Drawing for the job (mm, zero at the part's lowest x, y, z). A direction names the side the tool comes from. Coordinates: 2 decimals unless noted, no trailing zeros. Loops run counter-clockwise (first coordinate to the right, second up) from the corner with the lowest first, then second, coordinate; pieces in that order, holes last. Notation, with made-up numbers: (28.25, 8) -> (66.25, 8) arc R20 ccw to (66.25, 26) -> close; hole circle Ø1 at (72.25, -29). An arc over 180 degrees is marked (long way). Write each question's results on one line, items separated by ' | '.
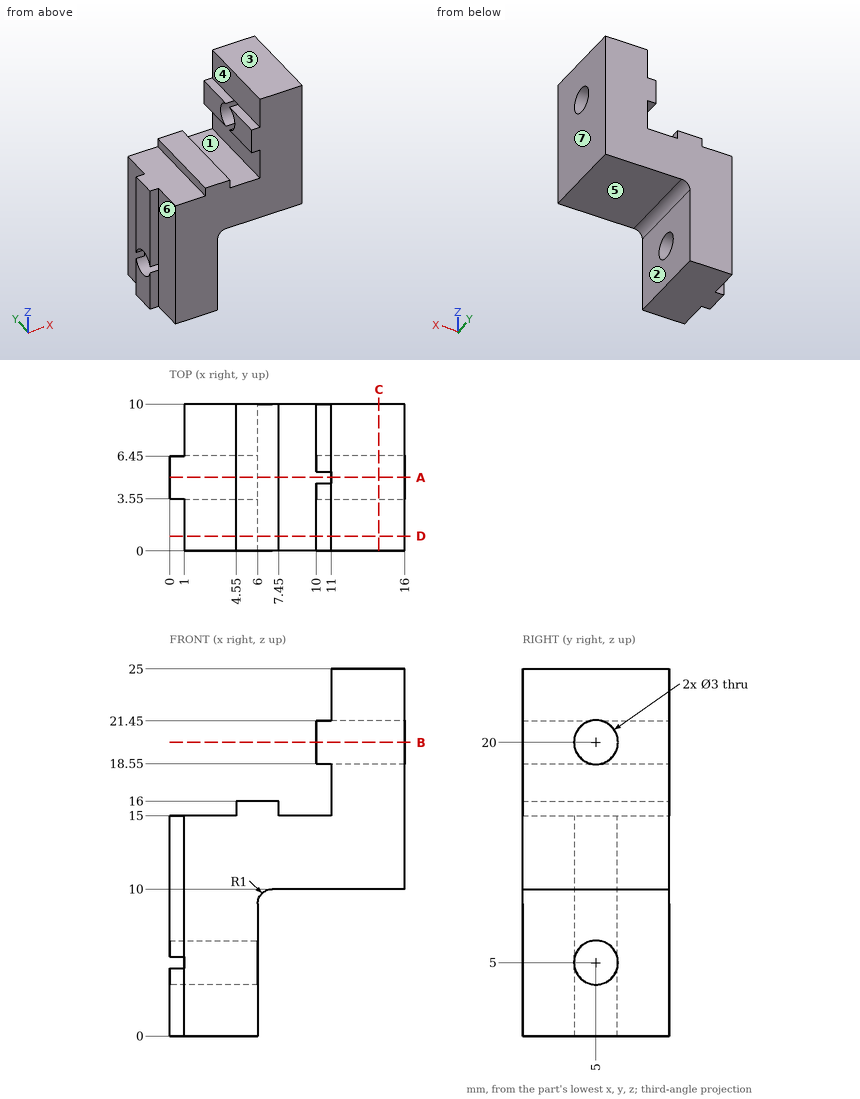
1) Slice it at D-D (y = 1). Write the cut outline in (x, z).
Outcome:
outline: (1, 0) -> (6, 0) -> (6, 9) arc R1 cw to (7, 10) -> (16, 10) -> (16, 25) -> (11, 25) -> (11, 21.45) -> (10, 21.45) -> (10, 18.55) -> (11, 18.55) -> (11, 15) -> (7.45, 15) -> (7.45, 16) -> (4.55, 16) -> (4.55, 15) -> (1, 15) -> close
2) Two-plate mould, pull along X, no slides. Class the marked faces 1, 2 and 3: pulls with the +X half, pulls with the -X half, needs draft (parallel to the pull), parting line crosses it, or undercut.
Outcome:
face 1: undercut | face 2: pulls with the +X half | face 3: needs draft
3) Drill centre lines: L1, parallel to Y at x = 12.7, z = 20; L2, parallel to Z at x = 3.65, y = 5; L3, parallel to Z at x = 14.15, y = 5. Where is each one in solid material? Low to high. Write a range as from..to.
Outcome:
L1: y = 0..3.5, 6.5..10 | L2: z = 0..3.5, 6.5..15 | L3: z = 10..18.5, 21.5..25
4) Which spindle directions (+Z, -Z, +X, -X, +Y, -Y) get a long thin tool onto all of the face, cutting with end or side? Do the marked faces 4, 5, 6 and 7. Say none if no direction does.
Outcome:
face 4: +Z, -X, +Y, -Y | face 5: -Z, +X, +Y, -Y | face 6: +Z, -Z, -X, -Y | face 7: +Z, -Z, +X, +Y, -Y
5) Slice it at A-A (y = 5). Write the cut outline in (x, z), then the cut area to 3 significant figures.
Outcome:
outline: (0, 0) -> (6, 0) -> (6, 3.5) -> (0, 3.5) -> close; (0, 6.5) -> (6, 6.5) -> (6, 9) arc R1 cw to (7, 10) -> (16, 10) -> (16, 18.5) -> (11, 18.5) -> (11, 15) -> (7.45, 15) -> (7.45, 16) -> (4.55, 16) -> (4.55, 15) -> (0, 15) -> close; (11, 21.5) -> (16, 21.5) -> (16, 25) -> (11, 25) -> close | area: 160 mm^2
6) Pin check, flat tips, straight feed: pin 1 (1.1 mm diameter, centred on y = 8, z = 6, fed in from -X); pin 2 (0.5 mm diameter, centred on x = 0.5, z = 12, fed in from -Y); pin 3 (1.8 mm diameter, centred on y = 5.5, z = 17.5, fed in from -X). Stop position of each tip, or through.
Outcome:
pin 1: stops at x = 1 | pin 2: stops at y = 3.55 | pin 3: stops at x = 11
7) Slice it at B-B (z = 20). Write the cut outline in (x, y), then the cut area to 3 significant figures.
Outcome:
outline: (10, 0) -> (16, 0) -> (16, 3.5) -> (10, 3.5) -> close; (10, 6.5) -> (16, 6.5) -> (16, 10) -> (10, 10) -> close | area: 42.0 mm^2
8) Slice it at C-C (x = 14.25). Write the cut outline in (y, z), then the cut area to 3 significant figures.
Outcome:
outline: (0, 10) -> (10, 10) -> (10, 25) -> (0, 25) -> close; hole circle Ø3 at (5, 20) | area: 143 mm^2
